Read the model definition and answer for the solid it produces. Units are mm, in the model's axes. Face numbers are marked on the shaded views. Round coordinates to 2 decimals unless told otherwise and drop trailing zeros. Order: outer loops, then holes, each group sorted by start corner. A loop starts at its lowest first (then second) coordinate and runs counter-clockwise, first axis right, second up. Notation, with made-up numbers: (15.25, 57.25) -> (40.25, 57.25) arc R23 ccw to (40.25, 87.25) -> close; hole circle Ø8 at (-12.5, -33). An arc over 180 degrees is marked (long way). One line per item, written item: value. Start each with the question number.
1. Flat-ended cylindrical pins translate along their axes: pin 1 Ø1.5 at (x, y) = (12, 3.5) entering from -Z; pin 2 Ø1.5 at (y, z) = (4, -4.5) entering from -X; pin 3 Ø3 at (x, z) = (28.5, 0) entering from +Y; pin 4 Ø1 at (y, z) = (3, -14.5) entering from -X. Find the tip coordinate at first contact, or state that the pin passes through.
2. Section B-B (x = 28.5) is taken. Give the vertices of the cut face in (y, z), then the cut area to 3 significant figures.
3. Section C-C (y = 3.3) is taken. Give the vertices of the cut face in (x, z).
4. Section D-D (x = 0) is taken. Give the vertices of the cut face in (y, z), then the cut area to 3 significant figures.
5. Section A-A (z = 4.5) is taken. Give the vertices of the cut face in (x, y).
6. The mould has two halves that part along X. Classify the marked faces 1, 2, 3 and 4: released by +X, released by -X, zero draft, split by the parting line, or undercut.
7. Consider line 1 (X direction, y = 2.25, z = 0); line 2 (Z direction, x = -30, y = 4); line 3 (X direction, y = 3.25, z = -17). Determine where each line is inside the solid, lowest interval first.
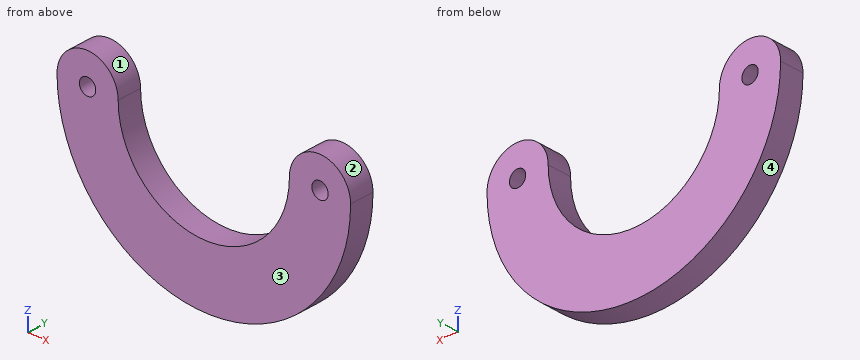
Autodesk Inventor part; units mm, degrees
ref_plane "YZ Plane" through (0, 0, 0) normal (1, 0, 0) x (0, 1, 0)
ref_plane "XZ Plane" through (0, 0, 0) normal (0, 1, 0) x (-1, 0, 0)
ref_plane "XY Plane" through (0, 0, 0) normal (0, 0, 1) x (1, 0, 0)
sketch "Sketch1" plane through (0, 0, 0) normal (0, 1, 0) x (-1, 0, 0)
  arc A0 (-21, 0) -> (21, 0) centre (0, 0) ccw
  arc A1 (-36, 0) -> (36, 0) centre (0, 0) ccw
  circle A2 centre (0, 0) radius 28.5
  circle A3 centre (28.5, 0) radius 2
  line L0 (0, 0) -> (36, 0) construction
  circle A4 centre (-28.5, 0) radius 2
  arc A5 (-21, 0) -> (-36, 0) centre (-28.5, 0) ccw
  arc A6 (36, 0) -> (21, 0) centre (28.5, 0) ccw
  dimension "d2" = 57
  dimension "d0" = 42
  dimension "d3" = 15
  dimension "d7" = 360
  dimension "d9" = 4
extrude "Extrusion1" add sketch "Sketch1" along normal blind 6 contours A0 A6 A2 A3 A4 A5 | A2 A4 A3 A6 A1 A5
properties part number "Mount" material "Plywood, Finish"
Answer:
1. pin 1: z = -34.2
1. pin 2: x = -35.8
1. pin 3: through
1. pin 4: x = -33.17
2. outline: (0, -21.99) -> (6, -21.99) -> (6, -2) -> (0, -2) -> close; (0, 2) -> (6, 2) -> (6, 7.5) -> (0, 7.5) -> close
2. area: 153 mm^2
3. outline: (-36, 0) arc R36 ccw to (36, 0) arc R7.5 ccw to (21, 0) arc R21 cw to (-21, 0) arc R7.5 ccw to start; hole circle Ø4 at (-28.5, 0); hole circle Ø4 at (28.5, 0)
4. outline: (0, -36) -> (6, -36) -> (6, -21) -> (0, -21) -> close
4. area: 90.0 mm^2
5. outline: (-34.5, 0) -> (-22.5, 0) -> (-22.5, 6) -> (-34.5, 6) -> close; (22.5, 0) -> (34.5, 0) -> (34.5, 6) -> (22.5, 6) -> close
6. face 1: undercut
6. face 2: undercut
6. face 3: zero draft
6. face 4: split by the parting line
7. line 1: -36 to -30.5, -26.5 to -21, 21 to 26.5, 30.5 to 36
7. line 2: -19.9 to -1.32, 1.32 to 7.35
7. line 3: -31.73 to -12.33, 12.33 to 31.73
